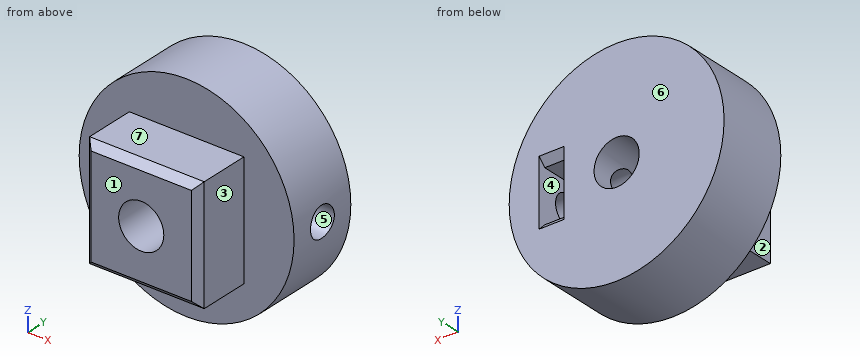
Autodesk Inventor part; units mm, degrees
ref_plane "YZ Plane" through (0, 0, 0) normal (1, 0, 0) x (0, 1, 0)
ref_plane "XZ Plane" through (0, 0, 0) normal (0, 1, 0) x (-1, 0, 0)
ref_plane "XY Plane" through (0, 0, 0) normal (0, 0, 1) x (1, 0, 0)
sketch "Boceto1" plane through (0, 0, 0) normal (0, 1, 0) x (-1, 0, 0)
  circle A0 centre (0, 0) radius 3.15
  circle A1 centre (0, 0) radius 15
  line L0 (-7.325, 3.6) -> (-10.825, 3.6)
  line L1 (-10.825, 3.6) -> (-10.825, -3.6)
  line L2 (-10.825, -3.6) -> (-7.325, -3.6)
  line L3 (-7.325, -3.6) -> (-7.325, 3.6)
  circle A2 centre (0, 0) radius 9.763 construction
  line L4 (6.7802, -4.5436) -> (0.5448, -8.1436)
  line L5 (8.5302, -7.5747) -> (6.7802, -4.5436)
  line L6 (2.2948, -11.1747) -> (8.5302, -7.5747)
  line L7 (0.5448, -8.1436) -> (2.2948, -11.1747)
  line L8 (0.5448, 8.1436) -> (6.7802, 4.5436)
  line L9 (2.2948, 11.1747) -> (0.5448, 8.1436)
  line L10 (8.5302, 7.5747) -> (2.2948, 11.1747)
  line L11 (6.7802, 4.5436) -> (8.5302, 7.5747)
  point P0 (-7.325, 0)
  point P1 (-9.075, 3.6)
  point P2 (3.6625, -6.3436)
  point P3 (1.4198, -9.6592)
  point P4 (3.6625, 6.3436)
  point P5 (7.6552, 6.0592)
  dimension "d0" = 6.3
  dimension "tuerca" = 7.2
  dimension "d2" = 11.85
  dimension "d3" = 6.613
  dimension "d4" = 3.5
  dimension "d18" = 360
  dimension "d26" = 30
  dimension "d27" = 4.175
  dimension "d28" = 4.175
extrude "Extrusión1" add sketch "Boceto1" along normal blind 10 contours A1 | L5 L6 L7 L4 | L9 L10 L11 L8
sketch "Boceto2" plane through (7.325, 0, -3.6) normal (1, 0, 0) x (0, 0, -1)
  line L0 (0, 0) -> (-7.2, 0)
  line L1 (0, 0) -> (0, 10) construction
  line L2 (-7.2, 10) -> (0, 10) construction
  line L3 (-7.2, 0) -> (-7.2, 10) construction
  line L4 (-7.2, 0) -> (0, 10) construction
  circle A0 centre (-3.6, 5) radius 2.1
  line L5 (0, 2.6906) -> (-4.6603, 0)
  line L6 (-2.5397, 0) -> (-7.2, 2.6906)
  line L7 (-7.2, 2.6906) -> (-7.2, 0)
  line L8 (0, 2.6906) -> (0, 0)
  point P0 (-3.6, 0)
  dimension "d7" = 4.2
  dimension "d8" = 120
  dimension "d9" = 3.8
extrude "Extrusión2" cut sketch "Boceto2" along normal mid plane 16 contours A0
extrude "Extrusión3" add sketch "Boceto2" along normal up to next contours L0 L6 L5 L8 | L0 L5 L6 | L0 L7 L6 L5
sketch "Boceto3" plane through (0, 0, 0) normal (0, -1, 0) x (1, 0, 0)
  circle A0 centre (0, 0) radius 3.15
  circle A1 centre (0, 0) radius 27.5
  line L0 (-8, 8) -> (8, 8)
  line L1 (8, 8) -> (8, -8)
  line L2 (8, -8) -> (-8, -8)
  line L3 (-8, -8) -> (-8, 8)
  point P0 (-8, 0)
  point P1 (0, 8)
  dimension "d32" = 16
  dimension "d33" = 55
extrude "Extrusión4" add sketch "Boceto3" along normal blind 8 contours L0 L1 L2 L3
chamfer "Chaflán1" distance 1 angle 45 2 edges at (9.075, 10, 3.6) (9.075, 10, -3.6)
chamfer "Chaflán3" distance 1 angle 45 4 edges at (0, -8, 8) (-8, -8, 0) (0, -8, -8) (8, -8, 0)
equation "\"d28\" = d27"
properties part number "dado polea"
The listing builds one solid part. Answer for the finished solid, in the listing's coordinates (mm). Face numbers are marked on the shaded views. A direction names the side the tool comes from. Coordinates: 2 decimals unless noted, no trailing zeros. Write each loop counter-clockwise with the first axis right and the second up, starting at its lowest first coordinate (ties: lowest second). Pieces come first, ordered by that corner, then holes.
Q1. Section A-A, the plane x = 0 is taken. Write down the section's boundary in (y, z), then the cut area to 3 significant figures.
Returned:
outline: (-8, -7) - (-7, -8) - (0, -8) - (0, -15) - (10, -15) - (10, -3.15) - (-8, -3.15) - close; (-8, 3.15) - (10, 3.15) - (10, 15) - (0, 15) - (0, 8) - (-7, 8) - (-8, 7) - close
area: 314 mm2
Q2. The mould has two halves that part along Z. Classify the marked faces 4, 5, 6 and 7: released by +Z, released by -Z, zero draft, split by the parting line, or undercut.
Returned:
face 4: undercut
face 5: undercut
face 6: zero draft
face 7: released by +Z
Q3. Find the intervals of material crossed by line 1 along X through (y, z) = (8.25, 0) (3 decimals); line 2 along X through (y, z) = (-3.75, 0); line 3 along Y through (x, z) = (4.25, 0), in increasing order.
Returned:
line 1: x = -15 to -3.15, 3.15 to 7.325, 10.825 to 15
line 2: x = -8 to -3.15, 3.15 to 8
line 3: y = -8 to 2.9, 7.1 to 10
Q4. Section B-B, the plane y = 8 is taken. Write down the section's boundary in (x, z) (3 decimals), then the cut area to 3 significant figures.
Returned:
outline: circle Ø30 at (0, 0); hole circle Ø6.3 at (0, 0); hole (7.325, -3.6) - (10.825, -3.6) - (10.825, 3.6) - (7.325, 3.6) - close
area: 650 mm2
Q5. Which of the six approach directions +Z, -Z, +X, -X, +Y, -Y give full straight-line access (tool end or side, diameter ignored) to the marked faces 1, 2 and 3?
Returned:
face 1: +Z, -Z, +X, -X, -Y
face 2: +Z, -Z, -X, -Y
face 3: +Z, -Z, +X, -Y
Q6. Section D-D, the plane y = -6.25 is taken. Write down the section's boundary in (x, z).
Returned:
outline: (-8, -8) - (8, -8) - (8, 8) - (-8, 8) - close; hole circle Ø6.3 at (0, 0)
Q7. Section C-C, the plane z = -2.5 is taken. Write down the section's boundary in (x, y) (3 decimals).
Returned:
outline: (-14.79, 0) - (-8, 0) - (-8, -7) - (-7, -8) - (-1.916, -8) - (-1.916, 10) - (-14.79, 10) - close; (1.916, -8) - (7, -8) - (8, -7) - (8, 0) - (14.79, 0) - (14.79, 10) - (10.825, 10) - (10.825, 2.056) - (7.325, 2.056) - (7.325, 10) - (1.916, 10) - close
Q8. Given P1, Ø6, axis at y = 0.5, z = 5, coming from the -X side; P2, Ø5, axis at x = 0, z = 0, coming from the -Y side; P3, Ø5, axis at x = -11.5, y = 1.5, coming from the +Z side; P4, Ø4, axis at y = 5, z = 0, coming from the +X side, each flat-ended and moving along its own axis, determine where each tip first touches the part or whether it passes through.
Returned:
P1: stops at x = -14.87
P2: passes through
P3: stops at z = 12
P4: stops at x = -2.43
